from build123d import *

# Parameters (mm, degrees)
F0_R          = 12.7
F1_DEPTH      = 17.78
F2_R          = 38.1
F3_DEPTH      = 10.16
F4_R          = 12.954
F5_DEPTH      = 17.781
F5_DEPTH_BACK = 115
F6_W          = 5.08
F6_H          = 45.466
F7_DEPTH      = 38.101
F7_DEPTH_BACK = 38.101
F8_W          = 38.608
F8_H          = 5.08
F9_DEPTH      = 38.101
F9_DEPTH_BACK = 38.101
F11_DEPTH     = 6.35


# Not quite as in the source:
# - an extrude ends at something that could not be found from the text; its depth is read off the source's solid


with BuildPart() as f1:
    # F0 (on Front) → F1 (new body)
    with BuildSketch(Plane.XZ):
        Circle(F0_R)
    extrude(amount=F1_DEPTH)

    # F2 (on Front) → F3 (join)
    with BuildSketch(Plane.XZ):
        Circle(F2_R)
    extrude(amount=F3_DEPTH)

    # F4 (on Front) → F5 (cut, two sides)
    with BuildSketch(Plane.XZ) as f5_sk:
        Circle(F4_R)
    extrude(amount=F5_DEPTH, mode=Mode.SUBTRACT)
    extrude(f5_sk.sketch, amount=-F5_DEPTH_BACK, mode=Mode.SUBTRACT)

    # F6 (on Right) → F7 (cut, two sides)
    with BuildSketch(Plane.YZ) as f7_sk:
        with Locations((-2.54, 0)):
            Rectangle(F6_W, F6_H)
    extrude(amount=F7_DEPTH, mode=Mode.SUBTRACT)
    extrude(f7_sk.sketch, amount=-F7_DEPTH_BACK, mode=Mode.SUBTRACT)

    # F8 (on Top) → F9 (cut, two sides)
    with BuildSketch(Plane.XY) as f9_sk:
        with Locations((0, -2.54)):
            Rectangle(F8_W, F8_H)
    extrude(amount=-F9_DEPTH, mode=Mode.SUBTRACT)
    extrude(f9_sk.sketch, amount=F9_DEPTH_BACK, mode=Mode.SUBTRACT)

    # F10 (on face) → F11 (cut)
    with BuildSketch(Plane(origin=(0, 0, 0), x_dir=(-1, 0, 0), z_dir=(0, 1, 0))):
        with BuildLine():
            Line((1.27, -1.27), (38.0788274504, -1.27))
            ThreePointArc((38.0788274504, -1.27), (38.1, 0), (38.0788274504, 1.27))
            Line((38.0788274504, 1.27), (1.27, 1.27))
            Line((1.27, 1.27), (1.27, 38.0788274504))
            ThreePointArc((1.27, 38.0788274504), (0, 38.1), (-1.27, 38.0788274504))
            Line((-1.27, 38.0788274504), (-1.27, 1.27))
            Line((-1.27, 1.27), (-38.0788274504, 1.27))
            ThreePointArc((-38.0788274504, 1.27), (-38.1, 0), (-38.0788274504, -1.27))
            Line((-38.0788274504, -1.27), (-1.27, -1.27))
            Line((-1.27, -1.27), (-1.27, -38.0788274504))
            ThreePointArc((-1.27, -38.0788274504), (0, -38.1), (1.27, -38.0788274504))
            Line((1.27, -38.0788274504), (1.27, -1.27))
        make_face()
    extrude(amount=-F11_DEPTH, mode=Mode.SUBTRACT)


solid = f1.part
Design review of the part built by this model. Coordinates are the model's own, in mm. A direction names the side the tool comes from. Coordinates: 2 decimals unless noted, no trailing zeros. Loops run counter-clockwise (first coordinate to the right, second up) from the corner with the lowest first, then second, coordinate; pieces in that order, holes last.
Item 1: Draft analysis for pull direction X (two halves, no side actions). For faces 1 (the flat face through (-24, 0, -27)), 2 (the flat face through (19.304, -3, -28)), 3 (the cylindrical face through (-28.08, -6.14, 25.75)), 4 (the flat face through (-16, -5.08, -16)), state which applies: pulls with the +X half, pulls with the -X half, needs draft (parallel to the pull), parting line crosses it, or undercut.
Completed:
face 1: needs draft
face 2: undercut
face 3: parting line crosses it
face 4: undercut
Item 2: Add section A-A (y = -3.75). Write out the cut boundary in (x, z).
Completed:
outline: (-30.57, -22.73) arc R38.1 ccw to (-19.3, -32.85) - (-19.3, -22.73) - close; (-30.57, 22.73) - (-19.3, 22.73) - (-19.3, 32.85) arc R38.1 ccw to start; (19.3, -32.85) arc R38.1 ccw to (30.57, -22.73) - (19.3, -22.73) - close; (19.3, 22.73) - (30.57, 22.73) arc R38.1 ccw to (19.3, 32.85) - close
Item 3: Add section D-D (y = -8). Write out the cut boundary in (x, z).
Completed:
outline: circle Ø76.2 at (0, 0); hole circle Ø25.91 at (0, 0)
Item 4: Clearance check with flat-ended pins moving along their axes: pin 1 (1.3 mm diameter, centred on x = 0, z = -31, fed in from +Y); pin 2 (5 mm diameter, centred on y = -8.5, z = 17, fed in from +X); pin 3 (2.5 mm diameter, centred on y = -3.5, z = 26.5, fed in from -X); pin 4 (1 mm diameter, centred on y = -4, z = -1, fed in from +X). State where each tip first meets the part, or that it passes through.
Completed:
pin 1: stops at y = -6.35
pin 2: stops at x = 35.23
pin 3: stops at x = -28.53
pin 4: passes through
Item 5: Wall thickness on L1, parallel to Z at x = 0, y = -6.4; L2, parallel to Y at x = 16, z = -14.5: over which ranges is each line inside the solid? List them lowest first.
Completed:
L1: z = -38.1 to -12.95, 12.95 to 38.1
L2: y = -10.16 to -5.08
Item 6: Add section B-B (x = 0). Write out the cut boundary in (y, z).
Completed:
outline: (-10.16, -38.1) - (-6.35, -38.1) - (-6.35, -12.95) - (-10.16, -12.95) - close; (-10.16, 12.95) - (-6.35, 12.95) - (-6.35, 38.1) - (-10.16, 38.1) - close
Item 7: Add section C-C (z = 0). Write out the cut boundary in (x, y), and give its area (3 significant figures).
Completed:
outline: (-38.1, -10.16) - (-12.95, -10.16) - (-12.95, -6.35) - (-38.1, -6.35) - close; (12.95, -10.16) - (38.1, -10.16) - (38.1, -6.35) - (12.95, -6.35) - close
area: 192 mm2
Item 8: For faces 5 (the flat face through (16, -10.16, 1)), 6 (the flat face through (26, -6.35, 0)), 7 (the flat face through (19.304, -3, 28)), list the 3-axis set-ups (+Z, -Z, +X, -X, +Y, -Y) from which the entire face can be reached by the end or side of a thin tool; tool diameter is ignored.
Completed:
face 5: +Z, -Z, +X, -X, -Y
face 6: +X, -X, +Y
face 7: +Z, -Z, +Y
